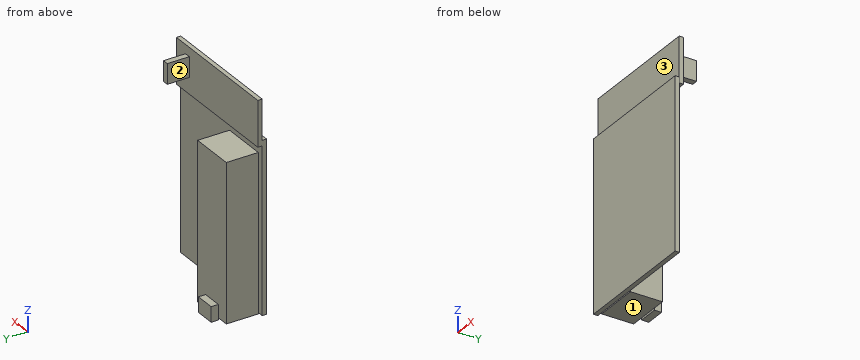
```python
from build123d import *

# Parameters (mm, degrees)
SKETCH1_W           = 50.165
SKETCH1_H           = 66.548
BOSS_EXTRUDE1_DEPTH = 1.7
SKETCH2_W           = 49.98833795
SKETCH2_H           = 17.78
BOSS_EXTRUDE2_DEPTH = 1.7
SKETCH3_W           = 17.6276
SKETCH3_H           = 61.2902
BOSS_EXTRUDE3_DEPTH = 12.5222
SKETCH4_W           = 7.8232
SKETCH4_H           = 5.9182
BOSS_EXTRUDE4_DEPTH = 2.794
SKETCH5_W           = 2.3368
SKETCH5_H           = 7.874
BOSS_EXTRUDE5_DEPTH = 8.636


with BuildPart() as part:
    # Sketch1 → Boss-Extrude1 (new body)
    with BuildSketch(Plane(origin=(0, 0, 0), x_dir=(1, 0, 0), z_dir=(0, 1, 0))):
        with Locations((-17.53077957, -2.078202509)):
            Rectangle(SKETCH1_W, SKETCH1_H)
    extrude(amount=BOSS_EXTRUDE1_DEPTH)

    # Sketch2 → Boss-Extrude2 (add)
    with BuildSketch(Plane(origin=(0, 1.7, 0), x_dir=(1, 0, 0), z_dir=(0, 1, 0))):
        with Locations((-17.619110595, -42.108602509)):
            Rectangle(SKETCH2_W, SKETCH2_H)
    extrude(amount=BOSS_EXTRUDE2_DEPTH)

    # Sketch3 → Boss-Extrude3 (add)
    with BuildSketch(Plane(origin=(0, 1.7, 0), x_dir=(1, 0, 0), z_dir=(0, 1, 0))):
        with Locations((-31.41187957, 1.058697491)):
            Rectangle(SKETCH3_W, SKETCH3_H)
    extrude(amount=BOSS_EXTRUDE3_DEPTH)

    # Sketch4 → Boss-Extrude4 (add)
    with BuildSketch(Plane(origin=(0, 14.2222, 0), x_dir=(1, 0, 0), z_dir=(0, 1, 0))):
        with Locations((-31.41187957, 29.582897491)):
            Rectangle(SKETCH4_W, SKETCH4_H)
    extrude(amount=BOSS_EXTRUDE4_DEPTH)

    # Sketch5 → Boss-Extrude5 (add)
    with BuildSketch(Plane(origin=(0, 3.4, 0), x_dir=(1, 0, 0), z_dir=(0, 1, 0))):
        with Locations((0.61865838, -43.531002509)):
            Rectangle(SKETCH5_W, SKETCH5_H)
    extrude(amount=BOSS_EXTRUDE5_DEPTH)


solid = part.part
```
Can you work these out from the model? Positions are in its coordinate system, mm. Face numbers are marked on the shaded views. A direction names the side the tool comes from. Round coordinates to 2 decimals unless told otherwise and drop trailing zeros. Order: outer loops, then holes, each group sorted by start corner. A loop starts at its lowest first (then second) coordinate and runs counter-clockwise, first axis right, second up. Notation, with made-up numbers: (-5.75, -31) -> (5.25, -31) arc R14 ccw to (5.25, -13) -> close; hole circle Ø2 at (43, 36.5). An arc over 180 degrees is marked (long way). Return JSON: item names as keys, results as strings. Group by question number.
1. Which directions (+Z, -Z, +X, -X, +Y, -Y) give clear straight access to the entire face, cutting with the end or side of a thin tool? Please do the marked faces 1, 2 and 3.
2. If we section it at A-A, the plane x = -36.5: Write out the boundary of the cut face in (y, z).
3. If we section it at C-C, the plane z = -20.5: Write out the boundary of the cut face in (x, y), then the cut area to 3 significant figures.
4. If we section it at B-B, the plane y = 10.5: Write out the boundary of the cut face in (x, z), then the cut area to 3 significant figures.
5. Will these pins go through, and if not, where does the flat tip stop? pin 1 (8 mm diameter, centred on y = 4.5, z = -9.5, fed in from -X); pin 2 (3 mm diameter, centred on y = 15, z = -29, fed in from +X); pin 3 (0.8 mm diameter, centred on y = 16, z = -29, fed in from -X); pin 4 (9 mm diameter, centred on x = -28.5, z = 7.5, fed in from +Y).
6. If we section it at D-D, the plane x = -20.5: Write out the boundary of the cut face in (y, z), then the cut area to 3 significant figures.
7. I need wall thicknesses on line 1 (Y direction, x = -21, z = -20); line 2 (Y direction, x = -39, z = -7); line 3 (X direction, y = 10.75, z = -10). Which ranges of each line are inside material? Lowest first, please. Write a range as [from, to].
Output values:
{
 "1": {"face 1": "-Z, +X, -X, -Y", "face 2": "+Z, -Z, -X, +Y", "face 3": "+Z, +X, -X, -Y"},
 "2": {"outline": "(0, -31.2) -> (1.7, -31.2) -> (1.7, -31.7) -> (14.22, -31.7) -> (14.22, 29.59) -> (1.7, 29.59) -> (1.7, 33.22) -> (3.4, 33.22) -> (3.4, 51) -> (1.7, 51) -> (1.7, 35.35) -> (0, 35.35) -> close"},
 "3": {"outline": "(-42.61, 0) -> (7.55, 0) -> (7.55, 1.7) -> (-22.6, 1.7) -> (-22.6, 14.22) -> (-40.23, 14.22) -> (-40.23, 1.7) -> (-42.61, 1.7) -> close", "area": "306 mm²"},
 "4": {"outline": "(-40.23, -31.7) -> (-22.6, -31.7) -> (-22.6, 29.59) -> (-40.23, 29.59) -> close; (-0.55, 39.59) -> (1.79, 39.59) -> (1.79, 47.47) -> (-0.55, 47.47) -> close", "area": "1,100 mm²"},
 "5": {"pin 1": "x = -42.61", "pin 2": "x = -22.6", "pin 3": "x = -35.32", "pin 4": "y = 14.22"},
 "6": {"outline": "(0, -31.2) -> (1.7, -31.2) -> (1.7, 33.22) -> (3.4, 33.22) -> (3.4, 51) -> (1.7, 51) -> (1.7, 35.35) -> (0, 35.35) -> close", "area": "143 mm²"},
 "7": {"line 1": "[0, 1.7]", "line 2": "[0, 14.22]", "line 3": "[-40.23, -22.6]"}
}
